from build123d import *

# Parameters (mm, degrees)
F0_R     = 4.15
F1_DEPTH = 3.5
F2_DEPTH = 10
F3_R     = 2.35
F4_DEPTH = 12.5794738247
F5_W     = 7.2
F5_H     = 3.2
F6_DEPTH = 8
F7_R     = 3


with BuildPart() as f1:
    # F0 (on Top) → F1 (new body)
    with BuildSketch(Plane.XY):
        with BuildLine():
            ThreePointArc((6, -4.5), (7.1151247354, -2.3717082451), (7.5, 0))
            ThreePointArc((7.5, 0), (-2.3717082451, 7.1151247354), (-6, -4.5))
            ThreePointArc((-6, -4.5), (0, -7.5), (6, -4.5))
        make_face()
        Circle(F0_R, mode=Mode.SUBTRACT)
    extrude(amount=F1_DEPTH)

    # F0 (on Top) → F2 (join)
    with BuildSketch(Plane.XY):
        with BuildLine():
            ThreePointArc((6, -4.5), (0, -7.5), (-6, -4.5))
            Line((-6, -4.5), (-6, -15))
            Line((-6, -15), (6, -15))
            Line((6, -15), (6, -4.5))
        make_face()
    extrude(amount=F2_DEPTH)

    # F3 (on face) → F4 (cut, up to face)
    with BuildSketch(Plane.XZ.offset(15)):
        with Locations((0, 3.815)):
            Circle(F3_R)
    extrude(amount=-F4_DEPTH, mode=Mode.SUBTRACT)

    # F5 (on face) → F6 (cut)
    with BuildSketch(Plane.XY):
        with Locations((0, -11.4)):
            Rectangle(F5_W, F5_H)
    extrude(amount=F6_DEPTH, mode=Mode.SUBTRACT)

    # F7
    f7_edges = [f1.edges().sort_by_distance(p)[0] for p in [
        (0, -7.5, 10),
    ]]
    fillet(f7_edges, radius=F7_R)


solid = f1.part
Can you work these out from the model? Positions are in its coordinate system, mm. A direction names the side the tool comes from. Round coordinates to 2 decimals unless told otherwise and drop trailing zeros. Write each loop counter-clockwise with the first axis right and the second up, starting at its lowest first coordinate (ties: lowest second). Pieces come first, ordered by that corner, then holes. Notation, with made-up numbers: (-7, 27) - (23, 27) arc R24 cw to (23, 62) - close; hole circle Ø8 at (65.5, 62.25). An arc over 180 degrees is marked (long way). Write each question's results on one line, items separated by ' | '. Start each with the question number.
1) Suppose I cut it at C-C (y = -12). List the corners of the cut face in (x, z) for me.
2) For pin 1 Ø3 at (x, y) = (-1.5, -11) entering from -Z; pin 2 Ø3 at (x, z) = (0, 3.815) entering from -Y; pin 3 Ø1.6 at (y, z) = (-12, 2.5) entering from -X; pin 4 Ø2.5 at (y, z) = (-11.5, 4) entering from +X, each with a flat end and sliding along its axis, tell me the tip position at first contact or that it passes through.
3) Which directions (+Z, -Z, +X, -X, +Y, -Y) give clear straight access to the entire face, cutting with the end or side of a thin tool? Please do faces 1 (the cylindrical face through (-0.51, -14.01, 1.52)), 2 (the flat face through (-2, -13, 6)), 3 (the cylindrical face through (0.1, -7.5, 6.4)).
4) We'd pull the mould along Z, two halves only. Please class faces 4 (the flat face through (0, -11, 8)), 5 (the flat face through (3, 4, 3.5)), 6 (the flat face through (-2, -9.8, 6)), 7 (the cylindrical face through (-0.51, -7.37, 1.52)): released by +Z, released by -Z, zero draft, split by the parting line, or undercut.
5) Suppose I cut it at B-B (z = 6.75). List the corners of the cut face in (x, y) for me.
6) Please list where these lines run through material, in increasing order: line 1 (Z direction, x = 0, y = -13.7) (3 decimals); line 2 (Z direction, x = 0.25, y = 5.5); line 3 (X direction, y = -11, z = 9.25).
7) Suppose I cut it at D-D (y = 3). List the corners of the cut face in (x, z) for me, and give its area (3 significant figures).
8) Suppose I cut it at A-A (x = 0). List the corners of the cut face in (y, z) for me (3 decimals).
Here are the results:
1) outline: (-6, 0) - (-3.6, 0) - (-3.6, 8) - (3.6, 8) - (3.6, 0) - (6, 0) - (6, 10) - (-6, 10) - close
2) pin 1: stops at z = 0 | pin 2: stops at y = 3.88 | pin 3: stops at x = -6 | pin 4: stops at x = 6
3) face 1: -Y | face 2: -Z | face 3: +Z, +Y
4) face 4: released by -Z | face 5: released by +Z | face 6: zero draft | face 7: undercut
5) outline: (-6, -15) - (6, -15) - (6, -4.5) arc R7.5 cw to (-6, -4.5) - close; hole (-3.6, -13) - (3.6, -13) - (3.6, -9.8) - (-3.6, -9.8) - close
6) line 1: z = 0 to 1.465, 6.165 to 10 | line 2: z = 0 to 3.5 | line 3: x = -6 to 6
7) outline: (-6.87, 0) - (-2.87, 0) - (-2.87, 3.5) - (-6.87, 3.5) - close; (2.87, 0) - (6.87, 0) - (6.87, 3.5) - (2.87, 3.5) - close | area: 28.0 mm2
8) outline: (-15, 0) - (-13, 0) - (-13, 1.465) - (-15, 1.465) - close; (-15, 6.165) - (-13, 6.165) - (-13, 8) - (-9.8, 8) - (-9.8, 6.165) - (-7.5, 6.165) - (-7.5, 7) arc R3 ccw to (-10.5, 10) - (-15, 10) - close; (-9.8, 0) - (-4.15, 0) - (-4.15, 1.465) - (-9.8, 1.465) - close; (4.15, 0) - (7.5, 0) - (7.5, 3.5) - (4.15, 3.5) - close
